```python
from build123d import *

# Parameters (mm, degrees)
SKETCH1_W           = 25.4
SKETCH1_H           = 25.4
SKETCH1_W_2         = 19.05
SKETCH1_H_2         = 19.05
BOSS_EXTRUDE1_DEPTH = 95.25
SKETCH2_R           = 2.4892
CUT_EXTRUDE1_DEPTH  = 95.25
SKETCH5_R           = 2.4892
CUT_EXTRUDE3_DEPTH  = 95.25


with BuildPart() as part:
    # Sketch1 → Boss-Extrude1 (new body)
    with BuildSketch(Plane.XY):
        with Locations((12.7, 12.7)):
            Rectangle(SKETCH1_W, SKETCH1_H)
        with Locations((12.7, 12.7)):
            Rectangle(SKETCH1_W_2, SKETCH1_H_2, mode=Mode.SUBTRACT)
    extrude(amount=BOSS_EXTRUDE1_DEPTH)

    # Sketch2 → Cut-Extrude1 (cut)
    with BuildSketch(Plane.ZY):
        with Locations((82.55, 14.2875)):
            Circle(SKETCH2_R)
        with Locations((69.85, 14.2875)):
            Circle(SKETCH2_R)
        with Locations((57.15, 14.2875)):
            Circle(SKETCH2_R)
        with Locations((44.45, 14.2875)):
            Circle(SKETCH2_R)
        with Locations((31.75, 14.2875)):
            Circle(SKETCH2_R)
        with Locations((19.05, 14.2875)):
            Circle(SKETCH2_R)
        with Locations((6.35, 14.2875)):
            Circle(SKETCH2_R)
    extrude(amount=-CUT_EXTRUDE1_DEPTH, mode=Mode.SUBTRACT)

    # Sketch5 → Cut-Extrude3 (cut)
    with BuildSketch(Plane(origin=(0, 0, 0), x_dir=(-1, 0, 0), z_dir=(0, -1, 0))):
        with Locations(Location((-12.7, -88.9, 0), (0, 0, 90))):
            Circle(SKETCH5_R)
        with Locations(Location((-12.7, -68.326, 0), (0, 0, 90))):
            Circle(SKETCH5_R)
        with Locations(Location((-12.7, -47.752, 0), (0, 0, 90))):
            Circle(SKETCH5_R)
        with Locations(Location((-12.7, -27.178, 0), (0, 0, 90))):
            Circle(SKETCH5_R)
        with Locations(Location((-12.7, -6.604, 0), (0, 0, 90))):
            Circle(SKETCH5_R)
    extrude(amount=-CUT_EXTRUDE3_DEPTH, mode=Mode.SUBTRACT)


solid = part.part
```
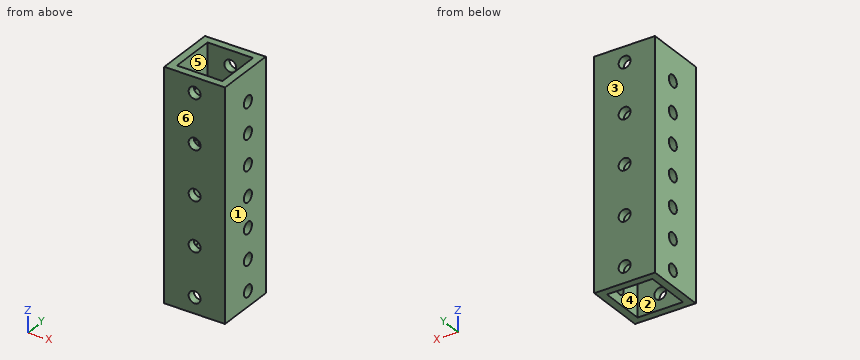
Design review of the part built by this model. Coordinates are the model's own, in mm. Face numbers are marked on the shaded views. A direction names the side the tool comes from. Give positions to 0.01 mm unless a question says otherwise; leave off trailing zeros. Order: outer loops, then holes, each group sorted by start corner. A loop starts at its lowest first (then second) coordinate and runs counter-clockwise, first axis right, second up. Notation, with made-up numbers: M 65,40 L 123,40 A12 cw 123,44 Z; hole C 77.5,6.5 d7. An arc over 180 degrees is marked long. One line per question, with ' | ' between items. Start each with the question number.
Q1. We need section B-B (x = 6.25). Write out the cut boundary in (y, z) (3 decimals), plus the area to 3 significant figures.
Q2. For pin 1 Ø8 at (x, z) = (12.7, 6.604) entering from +Y, flat-tipped, find the tip position at first contact; note if it passes through.
Q3. The part is to be moulded in two halves that separate along X. For the marked faces 1, 2, 3 and 4, say which applies: +X half, -X half, draft (parallel to the pull), parting line (faces both ways), or undercut.
Q4. For L1, parallel to Y at x = 24.25, z = 31.75; L2, parallel to Y at x = 3.5, z = 29 (3 decimals), list the stretches that pass through material, from the lowest coordinate up. Write a range as [from, to].
Q5. Machinability: for the marked faces 5 and 6, which of the approach directions +Z, -Z, +X, -X, +Y, -Y give a long, thin tool a straight path to every point of the face, cutting with its end or side? Answer none if there is none.
Q6. We need section D-D (z = 6.35). Write out the cut boundary in (x, y) (3 decimals), plus the area to 3 significant figures.
Q7. We need section A-A (z = 19.05). Write out the cut boundary in (x, y) (3 decimals), plus the area to 3 significant figures.
Returned:
1) outline: M 0,0 L 3.175,0 L 3.175,95.25 L 0,95.25 Z; M 22.225,0 L 25.4,0 L 25.4,95.25 L 22.225,95.25 Z | area: 605 mm2
2) pin 1: y = 25.4
3) face 1: +X half | face 2: undercut | face 3: draft | face 4: undercut
4) L1: [0, 11.8], [16.78, 25.4] | L2: [0, 3.175], [22.225, 25.4]
5) face 5: +Z, -Z | face 6: +Z, -Z, +X, -X, -Y
6) outline: M 0,0 L 10.224,0 L 10.224,3.175 L 3.175,3.175 L 3.175,11.798 L 0,11.798 Z; M 0,16.777 L 3.175,16.777 L 3.175,22.225 L 10.224,22.225 L 10.224,25.4 L 0,25.4 Z; M 15.176,0 L 25.4,0 L 25.4,11.798 L 22.225,11.798 L 22.225,3.175 L 15.176,3.175 Z; M 15.176,22.225 L 22.225,22.225 L 22.225,16.777 L 25.4,16.777 L 25.4,25.4 L 15.176,25.4 Z | area: 219 mm2
7) outline: M 0,0 L 25.4,0 L 25.4,11.798 L 22.225,11.798 L 22.225,3.175 L 3.175,3.175 L 3.175,11.798 L 0,11.798 Z; M 0,16.777 L 3.175,16.777 L 3.175,22.225 L 22.225,22.225 L 22.225,16.777 L 25.4,16.777 L 25.4,25.4 L 0,25.4 Z | area: 251 mm2
